The listing builds one solid part. Answer for the finished solid, in the listing's coordinates (mm). A direction names the side the tool comes from. Coordinates: 2 decimals unless noted, no trailing zeros. Answer in a Markdown table with one row per item.
```python
from build123d import *

# Parameters (mm, degrees)
SKETCH_1_R           = 80
EXTRUDE_1_DEPTH      = 20
SKETCH_2_R           = 23
SKETCH_2_R_2         = 17
CUT_EXTRUDE_1_DEPTH  = 8
SKETCH_3_R           = 38
SKETCH_3_R_2         = 32
CUT_EXTRUDE_2_DEPTH  = 8
SKETCH_4_R           = 53
SKETCH_4_R_2         = 47
CUT_EXTRUDE_3_DEPTH  = 8
SKETCH_5_R           = 68
SKETCH_5_R_2         = 62
CUT_EXTRUDE_4_DEPTH  = 8
SKETCH_6_R           = 1
CUT_EXTRUDE_5_DEPTH  = 12
SKETCH_7_R           = 1
CUT_EXTRUDE_6_DEPTH  = 12
SKETCH_8_R           = 1
CUT_EXTRUDE_7_DEPTH  = 12
SKETCH_9_R           = 0.75
CUT_EXTRUDE_8_DEPTH  = 12
SKETCH_10_R          = 3
CUT_EXTRUDE_9_DEPTH  = 161
SKETCH_11_R          = 2
CUT_EXTRUDE_10_DEPTH = 6
SKETCH_12_R          = 4.25
CUT_EXTRUDE_11_DEPTH = 161
CHAMFER_1_SIZE       = 1


with BuildPart() as part:
    # 草图1 → 凸台-拉伸1 (new body)
    with BuildSketch(Plane.XY):
        Circle(SKETCH_1_R)
    extrude(amount=EXTRUDE_1_DEPTH)

    # 草图2 → 切除-拉伸1 (cut)
    with BuildSketch(Plane.XY):
        Circle(SKETCH_2_R)
        Circle(SKETCH_2_R_2, mode=Mode.SUBTRACT)
    extrude(amount=CUT_EXTRUDE_1_DEPTH, mode=Mode.SUBTRACT)

    # 草图3 → 切除-拉伸2 (cut)
    with BuildSketch(Plane.XY):
        Circle(SKETCH_3_R)
        Circle(SKETCH_3_R_2, mode=Mode.SUBTRACT)
    extrude(amount=CUT_EXTRUDE_2_DEPTH, mode=Mode.SUBTRACT)

    # 草图4 → 切除-拉伸3 (cut)
    with BuildSketch(Plane.XY):
        Circle(SKETCH_4_R)
        Circle(SKETCH_4_R_2, mode=Mode.SUBTRACT)
    extrude(amount=CUT_EXTRUDE_3_DEPTH, mode=Mode.SUBTRACT)

    # 草图5 → 切除-拉伸4 (cut)
    with BuildSketch(Plane.XY):
        Circle(SKETCH_5_R)
        Circle(SKETCH_5_R_2, mode=Mode.SUBTRACT)
    extrude(amount=CUT_EXTRUDE_4_DEPTH, mode=Mode.SUBTRACT)

    # 草图6 → 切除-拉伸5 (cut)
    with BuildSketch(Plane.XY.offset(8)):
        with Locations((20, 0)):
            Circle(SKETCH_6_R)
        with Locations((14.142136, 14.142136)):
            Circle(SKETCH_6_R)
        with Locations((0, 20)):
            Circle(SKETCH_6_R)
        with Locations((-14.142136, 14.142136)):
            Circle(SKETCH_6_R)
        with Locations((-20, 0)):
            Circle(SKETCH_6_R)
        with Locations((-14.142136, -14.142136)):
            Circle(SKETCH_6_R)
        with Locations((0, -20)):
            Circle(SKETCH_6_R)
        with Locations((14.142136, -14.142136)):
            Circle(SKETCH_6_R)
    extrude(amount=CUT_EXTRUDE_5_DEPTH, mode=Mode.SUBTRACT)

    # 草图7 → 切除-拉伸6 (cut)
    with BuildSketch(Plane.XY.offset(8)):
        with Locations((34.327485, 6.828161)):
            Circle(SKETCH_7_R)
        with Locations((29.101436, 19.444958)):
            Circle(SKETCH_7_R)
        with Locations((19.444958, 29.101436)):
            Circle(SKETCH_7_R)
        with Locations((6.828161, 34.327485)):
            Circle(SKETCH_7_R)
        with Locations((-6.828161, 34.327485)):
            Circle(SKETCH_7_R)
        with Locations((-19.444958, 29.101436)):
            Circle(SKETCH_7_R)
        with Locations((-29.101436, 19.444958)):
            Circle(SKETCH_7_R)
        with Locations((-34.327485, 6.828161)):
            Circle(SKETCH_7_R)
        with Locations((-34.327485, -6.828161)):
            Circle(SKETCH_7_R)
        with Locations((-29.101436, -19.444958)):
            Circle(SKETCH_7_R)
        with Locations((-19.444958, -29.101436)):
            Circle(SKETCH_7_R)
        with Locations((-6.828161, -34.327485)):
            Circle(SKETCH_7_R)
        with Locations((6.828161, -34.327485)):
            Circle(SKETCH_7_R)
        with Locations((19.444958, -29.101436)):
            Circle(SKETCH_7_R)
        with Locations((29.101436, -19.444958)):
            Circle(SKETCH_7_R)
        with Locations((34.327485, -6.828161)):
            Circle(SKETCH_7_R)
    extrude(amount=CUT_EXTRUDE_6_DEPTH, mode=Mode.SUBTRACT)

    # 草图8 → 切除-拉伸7 (cut)
    with BuildSketch(Plane.XY.offset(8)):
        with Locations((50, 0)):
            Circle(SKETCH_8_R)
        with Locations((48.296291, 12.940952)):
            Circle(SKETCH_8_R)
        with Locations((43.30127, 25)):
            Circle(SKETCH_8_R)
        with Locations((35.355339, 35.355339)):
            Circle(SKETCH_8_R)
        with Locations((25, 43.30127)):
            Circle(SKETCH_8_R)
        with Locations((12.940952, 48.296291)):
            Circle(SKETCH_8_R)
        with Locations((0, 50)):
            Circle(SKETCH_8_R)
        with Locations((-12.940952, 48.296291)):
            Circle(SKETCH_8_R)
        with Locations((-25, 43.30127)):
            Circle(SKETCH_8_R)
        with Locations((-35.355339, 35.355339)):
            Circle(SKETCH_8_R)
        with Locations((-43.30127, 25)):
            Circle(SKETCH_8_R)
        with Locations((-48.296291, 12.940952)):
            Circle(SKETCH_8_R)
        with Locations((-50, 0)):
            Circle(SKETCH_8_R)
        with Locations((-48.296291, -12.940952)):
            Circle(SKETCH_8_R)
        with Locations((-43.30127, -25)):
            Circle(SKETCH_8_R)
        with Locations((-35.355339, -35.355339)):
            Circle(SKETCH_8_R)
        with Locations((-25, -43.30127)):
            Circle(SKETCH_8_R)
        with Locations((-12.940952, -48.296291)):
            Circle(SKETCH_8_R)
        with Locations((0, -50)):
            Circle(SKETCH_8_R)
        with Locations((12.940952, -48.296291)):
            Circle(SKETCH_8_R)
        with Locations((25, -43.30127)):
            Circle(SKETCH_8_R)
        with Locations((35.355339, -35.355339)):
            Circle(SKETCH_8_R)
        with Locations((43.30127, -25)):
            Circle(SKETCH_8_R)
        with Locations((48.296291, -12.940952)):
            Circle(SKETCH_8_R)
    extrude(amount=CUT_EXTRUDE_7_DEPTH, mode=Mode.SUBTRACT)

    # 草图9 → 切除-拉伸8 (cut)
    with BuildSketch(Plane.XY.offset(8)):
        with Locations((64.687007, 6.371114)):
            Circle(SKETCH_9_R)
        with Locations((62.201122, 18.868504)):
            Circle(SKETCH_9_R)
        with Locations((57.324882, 30.640788)):
            Circle(SKETCH_9_R)
        with Locations((50.245679, 41.235563)):
            Circle(SKETCH_9_R)
        with Locations((41.235563, 50.245679)):
            Circle(SKETCH_9_R)
        with Locations((30.640788, 57.324882)):
            Circle(SKETCH_9_R)
        with Locations((18.868504, 62.201122)):
            Circle(SKETCH_9_R)
        with Locations((6.371114, 64.687007)):
            Circle(SKETCH_9_R)
        with Locations((-6.371114, 64.687007)):
            Circle(SKETCH_9_R)
        with Locations((-18.868504, 62.201122)):
            Circle(SKETCH_9_R)
        with Locations((-30.640788, 57.324882)):
            Circle(SKETCH_9_R)
        with Locations((-41.235563, 50.245679)):
            Circle(SKETCH_9_R)
        with Locations((-50.245679, 41.235563)):
            Circle(SKETCH_9_R)
        with Locations((-57.324882, 30.640788)):
            Circle(SKETCH_9_R)
        with Locations((-62.201122, 18.868504)):
            Circle(SKETCH_9_R)
        with Locations((-64.687007, 6.371114)):
            Circle(SKETCH_9_R)
        with Locations((-64.687007, -6.371114)):
            Circle(SKETCH_9_R)
        with Locations((-62.201122, -18.868504)):
            Circle(SKETCH_9_R)
        with Locations((-57.324882, -30.640788)):
            Circle(SKETCH_9_R)
        with Locations((-50.245679, -41.235563)):
            Circle(SKETCH_9_R)
        with Locations((-41.235563, -50.245679)):
            Circle(SKETCH_9_R)
        with Locations((-30.640788, -57.324882)):
            Circle(SKETCH_9_R)
        with Locations((-18.868504, -62.201122)):
            Circle(SKETCH_9_R)
        with Locations((-6.371114, -64.687007)):
            Circle(SKETCH_9_R)
        with Locations((6.371114, -64.687007)):
            Circle(SKETCH_9_R)
        with Locations((18.868504, -62.201122)):
            Circle(SKETCH_9_R)
        with Locations((30.640788, -57.324882)):
            Circle(SKETCH_9_R)
        with Locations((41.235563, -50.245679)):
            Circle(SKETCH_9_R)
        with Locations((50.245679, -41.235563)):
            Circle(SKETCH_9_R)
        with Locations((57.324882, -30.640788)):
            Circle(SKETCH_9_R)
        with Locations((62.201122, -18.868504)):
            Circle(SKETCH_9_R)
        with Locations((64.687007, -6.371114)):
            Circle(SKETCH_9_R)
    extrude(amount=CUT_EXTRUDE_8_DEPTH, mode=Mode.SUBTRACT)

    # 草图10 → 切除-拉伸9 (cut, symmetric)
    with BuildSketch(Plane.XY):
        Circle(SKETCH_10_R)
    extrude(amount=CUT_EXTRUDE_9_DEPTH, both=True, mode=Mode.SUBTRACT)

    # 草图11 → 切除-拉伸10 (cut)
    with BuildSketch(Plane.XY.offset(20)):
        with Locations((57.5, 0)):
            Circle(SKETCH_11_R)
    extrude(amount=-CUT_EXTRUDE_10_DEPTH, mode=Mode.SUBTRACT)

    # 草图12 → 切除-拉伸11 (cut, symmetric)
    with BuildSketch(Plane.XY):
        with Locations((70.029622, 18.764381)):
            Circle(SKETCH_12_R)
        with Locations((51.265242, 51.265242)):
            Circle(SKETCH_12_R)
        with Locations((18.764381, 70.029622)):
            Circle(SKETCH_12_R)
        with Locations((-18.764381, 70.029622)):
            Circle(SKETCH_12_R)
        with Locations((-51.265242, 51.265242)):
            Circle(SKETCH_12_R)
        with Locations((-70.029622, 18.764381)):
            Circle(SKETCH_12_R)
        with Locations((-70.029622, -18.764381)):
            Circle(SKETCH_12_R)
        with Locations((-51.265242, -51.265242)):
            Circle(SKETCH_12_R)
        with Locations((-18.764381, -70.029622)):
            Circle(SKETCH_12_R)
        with Locations((18.764381, -70.029622)):
            Circle(SKETCH_12_R)
        with Locations((51.265242, -51.265242)):
            Circle(SKETCH_12_R)
        with Locations((70.029622, -18.764381)):
            Circle(SKETCH_12_R)
    extrude(amount=CUT_EXTRUDE_11_DEPTH, both=True, mode=Mode.SUBTRACT)

    # 倒角1
    chamfer_1_edges = [part.edges().sort_by_distance(p)[0] for p in [
        (-80, 0, 20),
    ]]
    chamfer(chamfer_1_edges, length=CHAMFER_1_SIZE)


solid = part.part
```
(1) Which of the six approach directions +Z, -Z, +X, -X, +Y, -Y give full straight-line access (tool end or side, diameter ignored) to faces 1 (the cylindrical face through (17.535, -33.713, 3.944)), 2 (the cylindrical face through (-52.187, 47.116, 9.86)), 3 (the cylindrical face through (59.347, -0.766, 17.042))?
Check values:
| item | result |
|---|---|
| face 1 | -Z |
| face 2 | +Z, -Z |
| face 3 | +Z |
(2) For a pull along Y with two mould halves and no side action, classify faces 4 (the flat face through (-1, -16, 20)), 5 (the cylindrical face through (36.556, 57.338, 3.944)) as released by +Y, released by -Y, zero draft, split by the parting line, or undercut.
Check values:
| item | result |
|---|---|
| face 4 | zero draft |
| face 5 | undercut |
(3) A cutting plane is placed at A-A, the plane z = 2.5. Count the separate pieces of the cut face and the enclosed holes in it, then the cut area to 3 significant figures.
Check values:
| item | result |
|---|---|
| separate pieces | 5 |
| enclosed holes | 17 |
| area | 13,000 mm² |
(4) Find the intervals of material crossed by line 1 along Y through (x, z) = (0, 16.5); line 2 along X through (y, z) = (7, 18); line 3 along Y through (x, z) = (-13.5, 17), in increasing order. Write a range as from..to.
Check values:
| item | result |
|---|---|
| line 1 | -80..-51, -49..-21, -19..-3, 3..19, 21..49, 51..80 |
| line 2 | -79.69..-65.1, -64.28..-35.31, -33.34..33.34, 35.31..64.28, 65.1..79.69 |
| line 3 | -78.85..-49.13, -47.47..-14.91, -13.38..13.38, 14.91..47.47, 49.13..78.85 |
(5) Flat-ended cylindrical pins translate along their axes: pin 1 (1 mm diameter, centred on x = -33.5, z = 5.5, fed in from +Y); pin 2 (2.5 mm diameter, centred on x = -14.14, y = -14.14, fed in from -Z); pin 3 (5 mm diameter, centred on y = -3.5, z = 13, fed in from +X). Find the tip coordinate at first contact, or state that the pin passes through.
Check values:
| item | result |
|---|---|
| pin 1 | y = 72.88 |
| pin 2 | z = 8 |
| pin 3 | x = 79.99 |
